Could you check a few things on this model? Use its own coordinates, in mm. Face numbers are marked on the shaded views. A direction names the side the tool comes from. Give positions to 0.01 mm unless a question says otherwise; leave off trailing zeros. Loops run counter-clockwise (first coordinate to the right, second up) from the corner with the lowest first, then second, coordinate; pieces in that order, holes last. Notation, with made-up numbers: M -35.75,-32 L 0.25,-32 A15 cw 0.25,-19 Z; hole C 44,45 d10. An arc over 180 degrees is marked long. Use a Markdown table: item, result. Add a question column.
1) Will these pins go through, and if not, where does the flat tip stop? pin 1 Ø1 at (x, z) = (0, -0.5) entering from +Y; pin 2 Ø5 at (x, z) = (-0.5, 1.5) entering from -Y; pin 3 Ø3.5 at (x, y) = (0, -0.5) entering from +Z.
2) Which directions (+Z, -Z, +X, -X, +Y, -Y) give clear straight access to the entire face, cutting with the end or side of a thin tool? Please do the marked faces 4 and 5.
3) We'd pull the mould along Y, two halves only. Please class the marked faces 1, 2 and 3: +Y half, -Y half, draft (parallel to the pull), parting line (faces both ways), or undercut.
4) Suppose I cut it at C-C on z = -1.25. List the corners of the cut face in (x, y) for me, and give its area (3 significant figures).
5) If I drill on line 1 along Y through (x, z) = (0, -1.25); line 2 along Y through (x, z) = (-2.5, 1), over which ranges is the centre line in solid material (lowest first)? Write a range as [from, to].
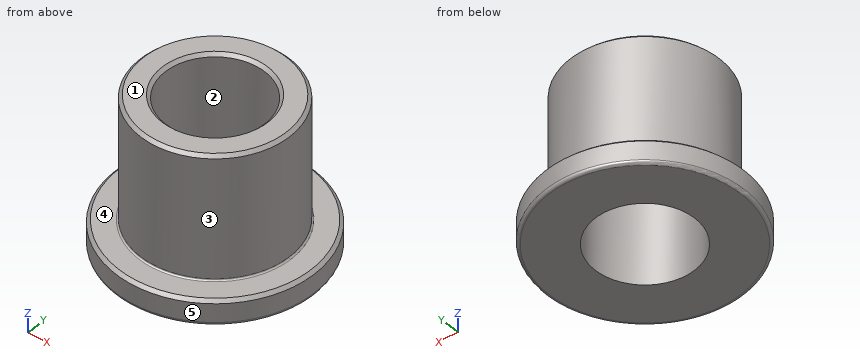
```python
from build123d import *

# Parameters (mm, degrees)
CHAMFER1_SIZE = 0.1984375
FILLET1_R     = 0.1984375
FILLET2_R     = 0.09921875


with BuildPart() as part:
    # Sketch3 → Revolve1 (revolve)
    with BuildSketch(Plane(origin=(0, 0, 0), x_dir=(0, 0, -1), z_dir=(1, 0, 0))):
        Polygon((4.7625, 6.35), (3.175, 6.35), (3.175, 4.7752), (-4.7625, 4.7752), (-4.7625, 3.1877), (4.7625, 3.1877), align=None)
    revolve(axis=Axis((0, 0, -4.7625), (0, 0, 1)))

    # Chamfer1
    chamfer1_edges = [part.edges().sort_by_distance(p)[0] for p in [
        (0, -3.1877, 4.7625),
        (0, -4.7752, 4.7625),
        (0, -6.35, -3.175),
    ]]
    chamfer(chamfer1_edges, length=CHAMFER1_SIZE)

    # Fillet1
    fillet1_edges = [part.edges().sort_by_distance(p)[0] for p in [
        (0, -6.35, -4.7625),
    ]]
    fillet(fillet1_edges, radius=FILLET1_R)

    # Fillet2
    fillet2_edges = [part.edges().sort_by_distance(p)[0] for p in [
        (0, -4.7752, -3.175),
    ]]
    fillet(fillet2_edges, radius=FILLET2_R)


solid = part.part
```
Answer block:
| question | item | result |
|---|---|---|
| 1 | pin 1 | stops at y = 4.78 |
| 1 | pin 2 | stops at y = -4.78 |
| 1 | pin 3 | passes through |
| 2 | face 4 | +Z |
| 2 | face 5 | +Z, -Z |
| 3 | face 1 | draft |
| 3 | face 2 | undercut |
| 3 | face 3 | parting line |
| 4 | outline | C 0,0 d9.55; hole C 0,0 d6.38 |
| 4 | area | 39.7 mm^2 |
| 5 | line 1 | y = [-4.78, -3.19], [3.19, 4.78] |
| 5 | line 2 | y = [-4.07, -1.98], [1.98, 4.07] |
